Build history of the part. All positions in model axes, mm. Face numbers are marked on the shaded views. A direction names the side the tool comes from. Give positions to 0.01 mm unless a question says otherwise; leave off trailing zeros. Loops run counter-clockwise (first coordinate to the right, second up) from the corner with the lowest first, then second, coordinate; pieces in that order, holes last. Notation, with made-up numbers: M 7,63 L 30,63 A20 ccw 30,75 Z; hole C 0,63.5 d9. An arc over 180 degrees is marked long. Answer in a Markdown table with one row per item. Add a question column.
```python
from build123d import *
from OCP.BRepFilletAPI import BRepFilletAPI_MakeFillet

# Parameters (mm, degrees)
BOSS_EXTRUDE1_DEPTH = 38.6
SKETCH4_W           = 12.7
SKETCH4_H           = 10
SKETCH4_W_2         = 8.3
SKETCH4_H_2         = 4.4
BOSS_EXTRUDE2_DEPTH = 0.35
FILLET1_R           = 0.5
SKETCH5_R           = 0.25
BOSS_EXTRUDE3_DEPTH = 0.1
CUT_EXTRUDE1_DEPTH  = 2
BOSS_EXTRUDE9_DEPTH = 14.2
CUT_EXTRUDE4_DEPTH  = 31.569586755
SKETCH7_W           = 10.1
SKETCH7_H           = 3.4
CUT_EXTRUDE2_DEPTH  = 43.050481162
BOSS_EXTRUDE5_DEPTH = 0.35
FILLET2_R1          = 0.5
FILLET2_R2          = 1
SKETCH9_R           = 0.25
BOSS_EXTRUDE6_DEPTH = 0.1
FILLET4_R           = 0.5
SKETCH16_W          = 0.1
SKETCH16_H          = 5.8
CUT_EXTRUDE6_DEPTH  = 0.1
SKETCH13_W          = 5.5
SKETCH13_H          = 7.5
CUT_EXTRUDE5_DEPTH  = 43.767974401
SKETCH14_W          = 0.5
SKETCH14_H          = 12.7
CUT_EXTRUDE7_DEPTH  = 11.3
SKETCH14_3_W        = 2.4
SKETCH14_3_H        = 9.7
SKETCH14_3_W_2      = 0.5
CUT_EXTRUDE8_DEPTH  = 5.3
CUT_EXTRUDE9_DEPTH  = 7.4
CUT_EXTRUDE10_START = -0.6
CUT_EXTRUDE10_DEPTH = 13


with BuildPart() as part:
    # Sketch2 → Boss-Extrude1 (new body)
    with BuildSketch(Plane.XY):
        with BuildLine():
            Line((0.965868705, -13.448021996), (0.965868705, -8.948021996))
            ThreePointArc((0.965868705, -8.948021996), (6.152703888, -6.568427123), (8.865868705, -1.548021996))
            Line((8.865868705, -1.548021996), (10.165868705, -1.548021996))
            Line((10.165868705, -1.548021996), (10.165868705, -13.448021996))
            Line((10.165868705, -13.448021996), (0.965868705, -13.448021996))
        make_face()
    extrude(amount=-BOSS_EXTRUDE1_DEPTH)

    # Sketch4 → Boss-Extrude2 (add)
    with BuildSketch(Plane(origin=(10.165868705, 0, 0), x_dir=(0, 0, -1), z_dir=(1, 0, 0))):
        with Locations((7.15, -7.248021996)):
            Rectangle(SKETCH4_W, SKETCH4_H)
        with Locations((19.35, -4.448021996)):
            Rectangle(SKETCH4_W_2, SKETCH4_H_2)
    extrude(amount=BOSS_EXTRUDE2_DEPTH)

    # Fillet1
    fillet1_edges = [part.edges().sort_by_distance(p)[0] for p in [
        (10.340868705, -2.248021996, -0.8),
        (10.340868705, -12.248021996, -0.8),
        (10.340868705, -12.248021996, -13.5),
        (10.340868705, -2.248021996, -13.5),
        (10.340868705, -2.248021996, -15.2),
        (10.340868705, -6.648021996, -15.2),
        (10.340868705, -6.648021996, -23.5),
        (10.340868705, -2.248021996, -23.5),
    ]]
    fillet(fillet1_edges, radius=FILLET1_R)

    # Sketch5 → Boss-Extrude3 (add)
    with BuildSketch(Plane(origin=(10.515868705, 0, 0), x_dir=(0, 0, -1), z_dir=(1, 0, 0))):
        with Locations(Location((1.3, -2.748021996, 0), (0, 0, 180))):
            Circle(SKETCH5_R)
        with Locations(Location((13, -2.748021996, 0), (0, 0, 180))):
            Circle(SKETCH5_R)
        with Locations((15.7, -2.748021996)):
            Circle(SKETCH5_R)
        with Locations((15.7, -6.148021996)):
            Circle(SKETCH5_R)
        with Locations(Location((13, -11.748021996, 0), (0, 0, 180))):
            Circle(SKETCH5_R)
        with Locations(Location((1.3, -11.748021996, 0), (0, 0, 180))):
            Circle(SKETCH5_R)
        with Locations((23, -2.748021996)):
            Circle(SKETCH5_R)
        with Locations((23, -6.148021996)):
            Circle(SKETCH5_R)
    extrude(amount=BOSS_EXTRUDE3_DEPTH)

    # Sketch3 → Cut-Extrude1 (cut)
    with BuildSketch(Plane(origin=(10.165868705, 0, 0), x_dir=(0, 0, -1), z_dir=(1, 0, 0))):
        Polygon((14.3, -13.448021996), (14.3, -7.348021996), (24.4, -7.348021996), (24.4, -1.548021996), (38.6, -1.548021996), (38.6, -13.448021996), align=None)
    extrude(amount=-CUT_EXTRUDE1_DEPTH, mode=Mode.SUBTRACT)

    # Sketch12 → Boss-Extrude9 (add)
    with BuildSketch(Plane(origin=(0, 0, -24.4), x_dir=(-1, 0, 0), z_dir=(0, 0, -1))):
        with BuildLine():
            Line((-8.165868705, -7.348021996), (-8.665868705, -7.348021996))
            Line((-8.665868705, -7.348021996), (-8.665868705, -15.048021996))
            Line((-8.665868705, -15.048021996), (-0.965868705, -15.048021996))
            Line((-0.965868705, -15.048021996), (-0.965868705, -8.948021996))
            ThreePointArc((-0.965868705, -8.948021996), (-4.526567846, -7.778829188), (-7.302349494, -5.260769133))
            ThreePointArc((-7.302349494, -5.260769133), (-7.689196636, -4.98209684), (-8.165868705, -4.991724772))
            Line((-8.165868705, -4.991724772), (-8.165868705, -7.348021996))
        make_face()
        with BuildLine():
            ThreePointArc((-8.165868705, -4.991724772), (-8.528297691, -5.266969628), (-8.665868705, -5.700776862))
            Line((-8.665868705, -5.700776862), (-8.665868705, -7.348021996))
            Line((-8.665868705, -7.348021996), (-8.165868705, -7.348021996))
            Line((-8.165868705, -7.348021996), (-8.165868705, -4.991724772))
        make_face()
    extrude(amount=BOSS_EXTRUDE9_DEPTH)

    # Sketch12<3> → Cut-Extrude4 (cut, through all)
    with BuildSketch(Plane(origin=(0, 0, -24.4), x_dir=(-1, 0, 0), z_dir=(0, 0, -1))):
        with BuildLine():
            Line((-8.165868705, -3.783991053), (-8.165868705, -4.991724772))
            ThreePointArc((-8.165868705, -4.991724772), (-7.689196636, -4.98209684), (-7.302349494, -5.260769133))
            ThreePointArc((-7.302349494, -5.260769133), (-7.769276796, -4.542943766), (-8.165868705, -3.783991053))
        make_face()
        with BuildLine():
            Line((-8.665868705, -2.429551313), (-8.665868705, -5.700776862))
            ThreePointArc((-8.665868705, -5.700776862), (-8.528297691, -5.266969628), (-8.165868705, -4.991724772))
            Line((-8.165868705, -4.991724772), (-8.165868705, -3.783991053))
            ThreePointArc((-8.165868705, -3.783991053), (-8.443072475, -3.116813627), (-8.665868705, -2.429551313))
        make_face()
    extrude(amount=CUT_EXTRUDE4_DEPTH, mode=Mode.SUBTRACT)

    # Sketch7 → Cut-Extrude2 (cut, through all)
    with BuildSketch(Plane(origin=(8.165868705, 0, 0), x_dir=(0, 0, -1), z_dir=(1, 0, 0))):
        with Locations((19.35, -11.748021996)):
            Rectangle(SKETCH7_W, SKETCH7_H)
    extrude(amount=-CUT_EXTRUDE2_DEPTH, mode=Mode.SUBTRACT)

    # Sketch8 → Boss-Extrude5 (add)
    with BuildSketch(Plane(origin=(8.665868705, 0, 0), x_dir=(0, 0, -1), z_dir=(1, 0, 0))):
        Polygon((25, -14.448021996), (25, -5.748021996), (37.7, -5.748021996), (37.7, -11.048021996), (34.3, -14.448021996), align=None)
    extrude(amount=BOSS_EXTRUDE5_DEPTH)

    # Fillet2: one fillet with a radius per group of edges: ONE call of the kernel's fillet builder (fillet() takes one radius for all edges)
    fillet2_edges_1 = [part.edges().sort_by_distance(p)[0] for p in [
        (8.840868705, -5.748021996, -25),
        (8.840868705, -14.448021996, -25),
        (8.840868705, -5.748021996, -37.7),
    ]]
    fillet2_edges_2 = [part.edges().sort_by_distance(p)[0] for p in [
        (8.840868705, -14.448021996, -34.3),
        (8.840868705, -11.048021996, -37.7),
    ]]
    fillet2 = BRepFilletAPI_MakeFillet(part.part.solid().wrapped)
    for e in fillet2_edges_1:
        fillet2.Add(FILLET2_R1, e.wrapped)
    for e in fillet2_edges_2:
        fillet2.Add(FILLET2_R2, e.wrapped)
    add(Compound.cast(fillet2.Shape()), mode=Mode.REPLACE)

    # Sketch9 → Boss-Extrude6 (add)
    with BuildSketch(Plane(origin=(9.015868705, 0, 0), x_dir=(0, 0, -1), z_dir=(1, 0, 0))):
        with Locations(Location((25.5, -6.248021996, 0), (0, 0, 180))):
            Circle(SKETCH9_R)
        with Locations(Location((25.5, -13.948021996, 0), (0, 0, 180))):
            Circle(SKETCH9_R)
        with Locations(Location((37.2, -6.248021996, 0), (0, 0, 180))):
            Circle(SKETCH9_R)
        with Locations(Location((34.092893219, -13.948021996, 0), (0, 0, 180))):
            Circle(SKETCH9_R)
        with Locations(Location((37.2, -10.840915215, 0), (0, 0, 180))):
            Circle(SKETCH9_R)
    extrude(amount=BOSS_EXTRUDE6_DEPTH)

    # Fillet4
    fillet4_edges = [part.edges().sort_by_distance(p)[0] for p in [
        (10.165868705, -13.448021996, -7.15),
        (10.165868705, -7.348021996, -19.35),
        (8.665868705, -15.048021996, -31.5),
        (8.165868705, -10.048021996, -19.35),
    ]]
    fillet(fillet4_edges, radius=FILLET4_R)

    # Sketch16 → Cut-Extrude6 (cut)
    with BuildSketch(Plane(origin=(10.165868705, 0, 0), x_dir=(0, 0, -1), z_dir=(1, 0, 0))):
        with Locations((14.35, -4.448021996)):
            Rectangle(SKETCH16_W, SKETCH16_H)
    extrude(amount=-CUT_EXTRUDE6_DEPTH, mode=Mode.SUBTRACT)

    # Sketch13 → Cut-Extrude5 (cut, through all)
    with BuildSketch(Plane(origin=(0, 0, 0), x_dir=(1, 0, 0), z_dir=(0, 1, 0))):
        with Locations((3.715868705, 12.25)):
            Rectangle(SKETCH13_W, SKETCH13_H)
    extrude(amount=-CUT_EXTRUDE5_DEPTH, mode=Mode.SUBTRACT)

    # Sketch14 → Cut-Extrude7 (cut)
    with BuildSketch(Plane(origin=(0, -1.548021996, 0), x_dir=(1, 0, 0), z_dir=(0, 1, 0))):
        Polygon((1.565868705, 1), (8.865868705, 1), (8.865868705, 13.7), (6.465868705, 13.7), (1.565868705, 13.7), align=None)
        with Locations((9.115868705, 7.35)):
            Rectangle(SKETCH14_W, SKETCH14_H)
    extrude(amount=-CUT_EXTRUDE7_DEPTH, mode=Mode.SUBTRACT)

    # Sketch14<3> → Cut-Extrude8 (cut)
    with BuildSketch(Plane(origin=(0, -1.548021996, 0), x_dir=(1, 0, 0), z_dir=(0, 1, 0))):
        with Locations((7.665868705, 18.55)):
            Rectangle(SKETCH14_3_W, SKETCH14_3_H)
        with Locations((9.115868705, 18.55)):
            Rectangle(SKETCH14_3_W_2, SKETCH14_3_H)
    extrude(amount=-CUT_EXTRUDE8_DEPTH, mode=Mode.SUBTRACT)

    # Sketch17 → Cut-Extrude9 (cut)
    with BuildSketch(Plane.XY.offset(-16)):
        with BuildLine():
            Line((6.465868705, -6.260394707), (6.465868705, -6.848021996))
            Line((6.465868705, -6.848021996), (5.839913933, -6.848021996))
            ThreePointArc((5.839913933, -6.848021996), (6.159902438, -6.561676764), (6.465868705, -6.260394707))
        make_face()
    extrude(amount=-CUT_EXTRUDE9_DEPTH, mode=Mode.SUBTRACT)

    # Sketch18 → Cut-Extrude10 (cut)
    with BuildSketch(Plane(origin=(0, 0, -38.6), x_dir=(-1, 0, 0), z_dir=(0, 0, -1)).offset(CUT_EXTRUDE10_START)):
        Polygon((-8.065868705, -14.448021996), (-8.065868705, -7.634559286), (-4.765868705, -7.634559286), (-4.765868705, -1.548021996), (-1.565868705, -1.548021996), (-1.565868705, -14.448021996), align=None)
    extrude(amount=-CUT_EXTRUDE10_DEPTH, mode=Mode.SUBTRACT)


solid = part.part
```
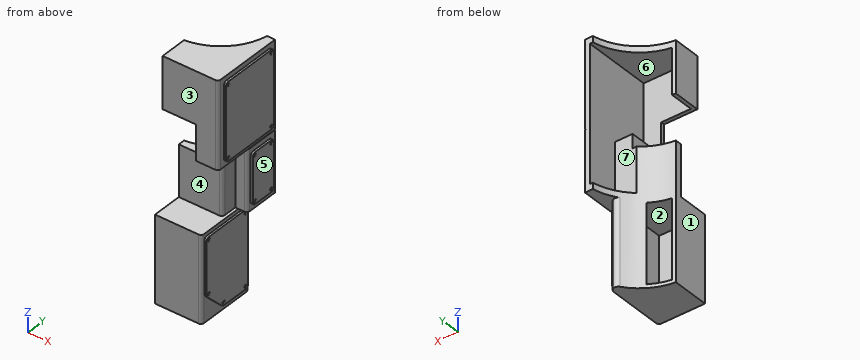
(1) Slice it at C-C, the plane y = -4.5. Give the cut face in (x, z), then the cut area to 3 significant figures.
(2) Slice it at D-D, the plane x = 2.5. Give the cut face in (y, z).
(3) Tool access for the marked faces 4, 5, 6 and 7: list every direction of +Z, -Z, +X, -X, +Y, -Y with a clear straight run to the whole face (end or side of a thin tool).
(4) Wall check: line 1 (Z direction, x = 2, y = -10.25); line 2 (Z direction, x = 4.25, y = -8.5); line 3 (X direction, y = -14, z = -35). Give the ranges that are in metal, low to high.
(5) Slice it at A-A, the plane x = 4.25. Give the cut face in (y, z).
(6) Slice it at B-B, the plane z = -9.5. Give the cut face in (x, y).
(7) Pull direction Y, two halves, no side cores. Call the marked faces 1, 2 and 3: +Y half, -Y half, draft (parallel to the pull), parting line (faces both ways), or undercut.
(8) Pin check, flat tips, straight feed: pin 1 (4 mm diameter, centred on y = -5.5, z = -13.5, fed in from +X); pin 2 (1 mm diameter, centred on x = 2.5, z = -34.5, fed in from +Y); pin 3 (2.5 mm diameter, centred on y = -9.5, z = -30, fed in from +X). Stop position of each tip, or through.
Solution:
| question | item | result |
|---|---|---|
| 1 | outline | M 7.79,-24.4 L 10.17,-24.4 L 10.17,-23.5 L 10.52,-23.5 L 10.52,-15.2 L 10.17,-15.2 L 10.17,-14.4 L 10.07,-14.4 L 10.07,-14.3 L 10.17,-14.3 L 10.17,-13.5 L 10.52,-13.5 L 10.52,-0.8 L 10.17,-0.8 L 10.17,0 L 7.79,0 L 7.79,-1 L 9.37,-1 L 9.37,-23.4 L 7.79,-23.4 Z |
| 1 | area | 30.0 mm^2 |
| 2 | outline | M -15.05,-38.6 L -8.65,-38.6 L -8.65,-38 L -14.45,-38 L -14.45,-25 L -8.65,-25 L -8.65,-16 L -10.05,-16 L -10.05,-24.4 L -15.05,-24.4 Z; M -13.45,-8.5 L -12.85,-8.5 L -12.85,-1 L -8.65,-1 L -8.65,0 L -13.45,0 Z |
| 3 | face 4 | +X, -X, -Y |
| 3 | face 5 | +X |
| 3 | face 6 | +Y |
| 3 | face 7 | -X, +Y |
| 4 | line 1 | -38.6 to -38, -25 to -24.4, -1 to 0 |
| 4 | line 2 | -38.6 to -38, -25 to -16, -1 to 0 |
| 4 | line 3 | 0.97 to 1.57, 8.07 to 8.67 |
| 5 | outline | M -15.05,-38.6 L -7.93,-38.6 L -7.93,-38 L -14.45,-38 L -14.45,-25 L -7.93,-25 L -7.93,-16 L -10.05,-16 L -10.05,-24.4 L -15.05,-24.4 Z; M -13.45,-8.5 L -12.85,-8.5 L -12.85,-1 L -7.93,-1 L -7.93,0 L -13.45,0 Z |
| 6 | outline | M 6.47,-13.45 L 9.67,-13.45 A0.5 ccw 10.17,-12.95 L 10.17,-12.25 L 10.52,-12.25 L 10.52,-2.25 L 10.17,-2.25 L 10.17,-1.55 L 9.37,-1.55 L 9.37,-12.85 L 6.47,-12.85 Z |
| 7 | face 1 | draft |
| 7 | face 2 | undercut |
| 7 | face 3 | -Y half |
| 8 | pin 1 | x = 10.52 |
| 8 | pin 2 | y = -14.45 |
| 8 | pin 3 | x = 9.02 |
